The model under review builds one solid part; all positions refer to its coordinate system, in mm. Coordinates: 2 decimals unless noted, no trailing zeros. Write each loop counter-clockwise with the first axis right and the second up, starting at its lowest first coordinate (ties: lowest second). Pieces come first, ordered by that corner, then holes. Notation, with made-up numbers: (-15, -2) - (20, -2) arc R20 cw to (20, 35) - close; hole circle Ø9 at (56.25, 2). An arc over 180 degrees is marked (long way). Put each result on its own line as item: value. Start each with the question number.
Item 1: Consider section B-B on y = 421.5. Give the boundary of the cut face in (x, z), then the cut area to 3 significant figures.
Item 2: To check wall thickness, follow L1, parallel to Y at x = 1.5, z = 11.25; L2, parallel to Z at x = 6.5, y = 328; L3, parallel to X at y = 592, z = 11.15. State the ranges of each line that lie inside material, in increasing order. Write a range as [from, to].
Item 3: Consider section A-A on z = 3.5. Give the boundary of the cut face in (x, y), then the cut area to 3 significant figures.
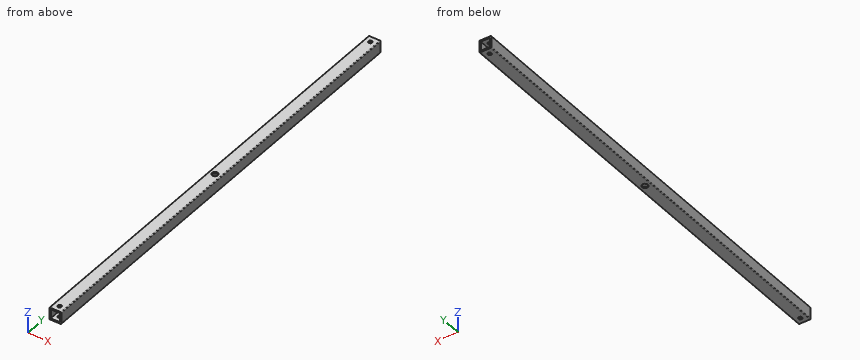
```python
from build123d import *

# Parameters (mm, degrees)
SKETCH1_W           = 16
SKETCH1_H           = 16
SKETCH1_W_2         = 12
SKETCH1_H_2         = 12
BOSS_EXTRUDE1_DEPTH = 600
FILLET1_R           = 1
SKETCH2_R           = 2.5
SKETCH2_R_2         = 4
CUT_EXTRUDE1_DEPTH  = 16


with BuildPart() as part:
    # Sketch1 → Boss-Extrude1 (new body)
    with BuildSketch(Plane(origin=(0, 0, 0), x_dir=(1, 0, 0), z_dir=(0, 1, 0))):
        with Locations((1.861111111, -3.916666667)):
            Rectangle(SKETCH1_W, SKETCH1_H)
        with Locations((1.861111111, -3.916666667)):
            Rectangle(SKETCH1_W_2, SKETCH1_H_2, mode=Mode.SUBTRACT)
    extrude(amount=BOSS_EXTRUDE1_DEPTH)

    # Fillet1
    fillet1_edges = [part.edges().sort_by_distance(p)[0] for p in [
        (-6.138888889, 300, -4.083333333),
        (9.861111111, 300, -4.083333333),
        (9.861111111, 300, 11.916666667),
        (-6.138888889, 300, 11.916666667),
    ]]
    fillet(fillet1_edges, radius=FILLET1_R)

    # Sketch2 → Cut-Extrude1 (cut)
    with BuildSketch(Plane(origin=(0, 0, -4.083333333), x_dir=(-1, 0, 0), z_dir=(0, 0, -1))):
        with Locations((-1.861111111, 8)):
            Circle(SKETCH2_R)
        with Locations((-1.861111111, 592)):
            Circle(SKETCH2_R)
        with Locations((-1.861111111, 300)):
            Circle(SKETCH2_R_2)
    extrude(amount=-CUT_EXTRUDE1_DEPTH, mode=Mode.SUBTRACT)


solid = part.part
```
Report:
1. outline: (-6.14, -3.08) arc R1 ccw to (-5.14, -4.08) - (8.86, -4.08) arc R1 ccw to (9.86, -3.08) - (9.86, 10.92) arc R1 ccw to (8.86, 11.92) - (-5.14, 11.92) arc R1 ccw to (-6.14, 10.92) - close; hole (-4.14, -2.08) - (7.86, -2.08) - (7.86, 9.92) - (-4.14, 9.92) - close
1. area: 111 mm²
2. L1: [0, 5.53], [10.47, 296.02], [303.98, 589.53], [594.47, 600]
2. L2: [-4.08, -2.08], [9.92, 11.92]
2. L3: [-6.11, -0.64], [4.36, 9.83]
3. outline: (-6.14, 0) - (-4.14, 0) - (-4.14, 600) - (-6.14, 600) - close; (7.86, 0) - (9.86, 0) - (9.86, 600) - (7.86, 600) - close
3. area: 2,400 mm²
